```python
from build123d import *

# Parameters (mm, degrees)
SKETCH1_W                = 9
SKETCH1_H                = 55
SKETCH1_W_2              = 91
SKETCH1_H_2              = 5
BOSS_EXTRUDE3_DEPTH      = 5
SKETCH6_W                = 18
SKETCH6_H                = 60
BOSS_EXTRUDE4_DEPTH      = 18
SKETCH7_W                = 91
SKETCH7_H                = 5
BOSS_EXTRUDE5_DEPTH      = 100
SKETCH13_W               = 18
SKETCH13_H               = 5
CUT_EXTRUDE6_DEPTH       = 75
SKETCH16_R               = 4.2
CUT_EXTRUDE7_DEPTH       = 20
CUT_EXTRUDE8_DEPTH       = 75
CUT_EXTRUDE10_DEPTH      = 8
CUT_EXTRUDE11_DEPTH      = 22
CUT_EXTRUDE14_DEPTH      = 34
CUT_EXTRUDE14_DEPTH_BACK = 5
FILLET4_R                = 10
CUT_EXTRUDE15_DEPTH      = 24
CUT_EXTRUDE15_DEPTH_BACK = 1
SKETCH23_R               = 19.425
SKETCH24_R               = 1.315
CUT_EXTRUDE16_DEPTH      = 10
SKETCH26_W               = 40
SKETCH26_H               = 5
BOSS_EXTRUDE6_DEPTH      = 10


with BuildPart() as part:
    # Sketch1 → Boss-Extrude3 (new body)
    with BuildSketch(Plane.XY):
        with Locations((41, -0.737170899)):
            Rectangle(SKETCH1_W, SKETCH1_H)
        with Locations((32, -0.737170899)):
            Rectangle(SKETCH1_W, SKETCH1_H)
        with BuildLine():
            Line((27.5, 26.762829101), (0, 26.762829101))
            Line((0, 26.762829101), (0, 10.762829101))
            ThreePointArc((0, 10.762829101), (8.131727984, 7.394557085), (11.5, -0.737170899))
            ThreePointArc((11.5, -0.737170899), (8.131727984, -8.868898883), (0, -12.237170899))
            Line((0, -12.237170899), (0, -28.237170899))
            Line((0, -28.237170899), (27.5, -28.237170899))
            Line((27.5, -28.237170899), (27.5, 26.762829101))
        make_face()
        with BuildLine():
            Line((0, 10.762829101), (0, 26.762829101))
            Line((0, 26.762829101), (-27.5, 26.762829101))
            Line((-27.5, 26.762829101), (-27.5, -28.237170899))
            Line((-27.5, -28.237170899), (0, -28.237170899))
            Line((0, -28.237170899), (0, -12.237170899))
            ThreePointArc((0, -12.237170899), (-11.5, -0.737170899), (0, 10.762829101))
        make_face()
        with Locations((-32, -0.737170899)):
            Rectangle(SKETCH1_W, SKETCH1_H)
        with Locations((-41, -0.737170899)):
            Rectangle(SKETCH1_W, SKETCH1_H)
        with Locations((0, 29.262829101)):
            Rectangle(SKETCH1_W_2, SKETCH1_H_2)
    extrude(amount=BOSS_EXTRUDE3_DEPTH)

    # Sketch6 → Boss-Extrude4 (add)
    with BuildSketch(Plane(origin=(0, 0, 0), x_dir=(-1, 0, 0), z_dir=(0, 0, -1))):
        with Locations((-36.5, 1.762829101)):
            Rectangle(SKETCH6_W, SKETCH6_H)
        with Locations((36.5, 1.762829101)):
            Rectangle(SKETCH6_W, SKETCH6_H)
    extrude(amount=BOSS_EXTRUDE4_DEPTH)

    # Sketch7 → Boss-Extrude5 (add)
    with BuildSketch(Plane.XY.offset(5)):
        with Locations((0, 29.262829101)):
            Rectangle(SKETCH7_W, SKETCH7_H)
    extrude(amount=BOSS_EXTRUDE5_DEPTH)

    # Sketch13 → Cut-Extrude6 (cut)
    with BuildSketch(Plane(origin=(0, 31.762829101, 0), x_dir=(1, 0, 0), z_dir=(0, 1, 0))):
        with Locations((-36.5, 15.5)):
            Rectangle(SKETCH13_W, SKETCH13_H)
        with Locations((36.5, 15.5)):
            Rectangle(SKETCH13_W, SKETCH13_H)
    extrude(amount=-CUT_EXTRUDE6_DEPTH, mode=Mode.SUBTRACT)

    # Sketch16 → Cut-Extrude7 (cut)
    with BuildSketch(Plane(origin=(0, 31.762829101, 0), x_dir=(1, 0, 0), z_dir=(0, 1, 0))):
        with Locations(Location((-36.5, 4, 0), (0, 0, 180))):
            Circle(SKETCH16_R)
        with Locations(Location((36.5, 4, 0), (0, 0, 180))):
            Circle(SKETCH16_R)
    extrude(amount=-CUT_EXTRUDE7_DEPTH, mode=Mode.SUBTRACT)

    # Sketch17 → Cut-Extrude8 (cut)
    with BuildSketch(Plane(origin=(0, 31.762829101, 0), x_dir=(1, 0, 0), z_dir=(0, 1, 0))):
        with BuildLine():
            Line((-45.5, 13), (-45.5, 4))
            ThreePointArc((-45.5, 4), (-42.863961031, 10.363961031), (-36.5, 13))
            Line((-36.5, 13), (-45.5, 13))
        make_face()
        with BuildLine():
            ThreePointArc((-36.5, 13), (-30.136038969, 10.363961031), (-27.5, 4))
            Line((-27.5, 4), (-27.5, 13))
            Line((-27.5, 13), (-36.5, 13))
        make_face()
        with BuildLine():
            Line((27.5, 13), (27.5, 4))
            ThreePointArc((27.5, 4), (30.136038969, 10.363961031), (36.5, 13))
            Line((36.5, 13), (27.5, 13))
        make_face()
        with BuildLine():
            Line((45.5, 13), (36.5, 13))
            ThreePointArc((36.5, 13), (42.863961031, 10.363961031), (45.5, 4))
            Line((45.5, 4), (45.5, 13))
        make_face()
    extrude(amount=-CUT_EXTRUDE8_DEPTH, mode=Mode.SUBTRACT)

    # Sketch18 → Cut-Extrude10 (cut)
    with BuildSketch(Plane(origin=(0, 31.762829101, 0), x_dir=(1, 0, 0), z_dir=(0, 1, 0))):
        with BuildLine():
            ThreePointArc((-45.5, -105), (-26.743051045, -83.063543967), (-20, -55))
            Line((-20, -55), (-45.5, -55))
            Line((-45.5, -55), (-45.5, -105))
        make_face()
        with BuildLine():
            Line((-45.5, -55), (-20, -55))
            ThreePointArc((-20, -55), (-26.743051045, -26.936456033), (-45.5, -5))
            Line((-45.5, -5), (-45.5, -55))
        make_face()
        with BuildLine():
            ThreePointArc((-45.5, -105), (-26.743051045, -83.063543967), (-20, -55))
            Line((-20, -55), (-45.5, -55))
            Line((-45.5, -55), (-45.5, -105))
        make_face()
        with BuildLine():
            Line((-45.5, -55), (-20, -55))
            ThreePointArc((-20, -55), (-26.743051045, -26.936456033), (-45.5, -5))
            Line((-45.5, -5), (-45.5, -55))
        make_face()
        with BuildLine():
            Line((-20, -105), (-20, -55))
            ThreePointArc((-20, -55), (-26.743051045, -83.063543967), (-45.5, -105))
            Line((-45.5, -105), (-20, -105))
        make_face()
        with BuildLine():
            Line((20, -55), (20, -105))
            Line((20, -105), (45.5, -105))
            ThreePointArc((45.5, -105), (26.743051045, -83.063543967), (20, -55))
        make_face()
        with BuildLine():
            Line((45.5, -55), (45.5, -5))
            ThreePointArc((45.5, -5), (26.743051045, -26.936456033), (20, -55))
            Line((20, -55), (45.5, -55))
        make_face()
        with BuildLine():
            ThreePointArc((20, -55), (26.743051045, -83.063543967), (45.5, -105))
            Line((45.5, -105), (45.5, -55))
            Line((45.5, -55), (20, -55))
        make_face()
        with BuildLine():
            Line((45.5, -55), (45.5, -5))
            ThreePointArc((45.5, -5), (26.743051045, -26.936456033), (20, -55))
            Line((20, -55), (45.5, -55))
        make_face()
        with BuildLine():
            ThreePointArc((20, -55), (26.743051045, -83.063543967), (45.5, -105))
            Line((45.5, -105), (45.5, -55))
            Line((45.5, -55), (20, -55))
        make_face()
    extrude(amount=-CUT_EXTRUDE10_DEPTH, mode=Mode.SUBTRACT)

    # Sketch19 → Cut-Extrude11 (cut)
    with BuildSketch(Plane.XY.offset(5)):
        with BuildLine():
            Line((-32.5, -0.737170899), (-45.5, -0.737170899))
            Line((-45.5, -0.737170899), (-45.5, -28.237170899))
            Line((-45.5, -28.237170899), (-17.320508076, -28.237170899))
            ThreePointArc((-17.320508076, -28.237170899), (-28.453176558, -16.442798673), (-32.5, -0.737170899))
        make_face()
        with BuildLine():
            Line((45.5, -28.237170899), (17.320508076, -28.237170899))
            ThreePointArc((17.320508076, -28.237170899), (28.453176558, -16.442798673), (32.5, -0.737170899))
            Line((32.5, -0.737170899), (45.5, -0.737170899))
            Line((45.5, -0.737170899), (45.5, -28.237170899))
        make_face()
    extrude(amount=-CUT_EXTRUDE11_DEPTH, mode=Mode.SUBTRACT)

    # Sketch21 → Cut-Extrude14 (cut, two sides: drawn at the far end of the back side and taken through both)
    with BuildSketch(Plane.XZ.offset(0.737170899).offset(-CUT_EXTRUDE14_DEPTH_BACK)):
        with BuildLine():
            Line((27.5, 0), (32.5, 0))
            Line((32.5, 0), (32.5, 5))
            Line((32.5, 5), (45.5, 5))
            Line((45.5, 5), (45.5, -4))
            ThreePointArc((45.5, -4), (36.5, -13), (27.5, -4))
            Line((27.5, -4), (27.5, 0))
        make_face()
        with BuildLine():
            Line((-27.5, -4), (-27.5, 0))
            Line((-27.5, 0), (-32.5, 0))
            Line((-32.5, 0), (-32.5, 5))
            Line((-32.5, 5), (-45.5, 5))
            Line((-45.5, 5), (-45.5, -4))
            ThreePointArc((-45.5, -4), (-36.5, -13), (-27.5, -4))
        make_face()
    extrude(amount=CUT_EXTRUDE14_DEPTH + CUT_EXTRUDE14_DEPTH_BACK, mode=Mode.SUBTRACT)

    # Fillet4
    # the kernel refuses this fillet: 10 mm, written as the material it adds along each edge
    with BuildSketch(Plane(origin=(70.5, 26.762829101, 5), x_dir=(0, -1, 0), z_dir=(-1, 0, 0))) as fillet4_piece_1_section:
        with BuildLine():
            CenterArc((FILLET4_R, FILLET4_R), FILLET4_R, 180, 90)
            Line((0, FILLET4_R), (0, 0))
            Line((0, 0), (FILLET4_R, 0))
        make_face()
    fillet4_piece_1 = extrude(amount=141, mode=Mode.PRIVATE)
    fillet4_piece_1 = fillet4_piece_1 - Plane(origin=(-81.769607843, 24.471447362, 55), x_dir=(0.5871756209824568, 0, 0.8094595667010591), z_dir=(0, 1, 0)) * Cylinder(61.769607843, 322, mode=Mode.PRIVATE)
    fillet4_piece_1 = fillet4_piece_1 - Plane(origin=(81.769607843, 24.471447362, 55), x_dir=(-0.5871756209824566, 0, -0.8094595667010592), z_dir=(0, 1, 0)) * Cylinder(61.769607843, 322, mode=Mode.PRIVATE)
    add(fillet4_piece_1)

    # Sketch23 → Cut-Extrude15 (cut, two sides: drawn at the far end of the back side and taken through both)
    with BuildSketch(Plane.XY.offset(5).offset(-CUT_EXTRUDE15_DEPTH_BACK)):
        with Locations(Location((0, -0.737170899, 0), (0, 0, 115.723259522))):
            Circle(SKETCH23_R)
    extrude(amount=CUT_EXTRUDE15_DEPTH + CUT_EXTRUDE15_DEPTH_BACK, mode=Mode.SUBTRACT)

    # Sketch24 → Cut-Extrude16 (cut)
    with BuildSketch(Plane.XY.offset(4)):
        with Locations((-8.4, 13.812055885)):
            Circle(SKETCH24_R)
        with Locations((8.4, -15.286397682)):
            Circle(SKETCH24_R)
        with Locations((-8.4, -15.286397682)):
            Circle(SKETCH24_R)
        with Locations((16.8, -0.737170899)):
            Circle(SKETCH24_R)
        with Locations((-16.8, -0.737170899)):
            Circle(SKETCH24_R)
        with Locations((8.4, 13.812055885)):
            Circle(SKETCH24_R)
    extrude(amount=-CUT_EXTRUDE16_DEPTH, mode=Mode.SUBTRACT)

    # Sketch26 → Boss-Extrude6 (add)
    with BuildSketch(Plane.XY.offset(105)):
        with Locations((0, 29.262829101)):
            Rectangle(SKETCH26_W, SKETCH26_H)
    extrude(amount=BOSS_EXTRUDE6_DEPTH)


solid = part.part
```
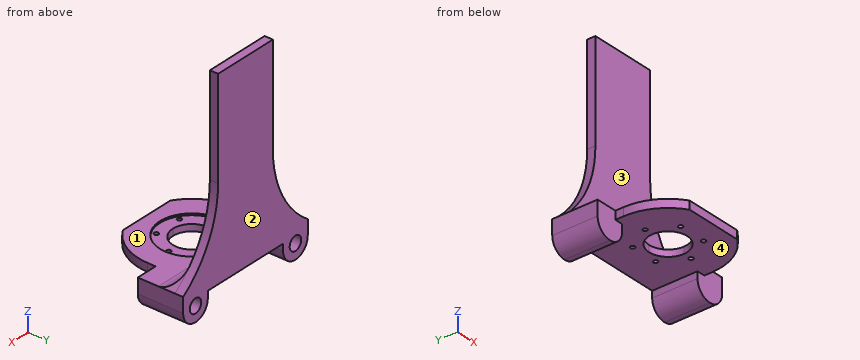
Check sheet for the modelled part. Datum: model origin and axes. Units: mm. Face numbers are marked on the shaded views. A direction names the side the tool comes from. Coordinates: 2 decimals unless noted, no trailing zeros. Loops run counter-clockwise (first coordinate to the right, second up) from the corner with the lowest first, then second, coordinate; pieces in that order, holes last.
1) Access from +Z, -Z, +X, -X, +Y, -Y to the whole of each face (thin tool, end or side, straight path). Record for the marked faces 1 and 2.
2) Sectioned sample at B-B (z = 104.5). Record the boundary of the cut face in (x, y).
3) Sectioned sample at C-C (y = 22). Record the boundary of the cut face in (x, z), and give its area (3 significant figures).
4) Release check for a two-part mould opening along X. For the marked faces 3 and 4 record: released by +X, released by -X, zero draft, split by the parting line, or undercut.
5) Gauge pin test, flat ends, axial feed: pin 1 (5 mm diameter, centred on x = -36.5, z = -4, fed in from -Y); pin 2 (2.5 mm diameter, centred on y = 2, z = 1.5, fed in from -X); pin 3 (3 mm diameter, centred on x = 4.5, y = 9.5, fed in from -Z). Record the tip position at first contact, or that the pin passes through.
6) Sectioned sample at A-A (y = 8). Record the boundary of the cut face in (x, z).
7) Material ranges on probe 1 along Y at (x, z) = (0, 4.75); probe 2 along Y at (x, z) = (16.8, 1.3); probe 3 along Z at (x, y) = (36, 16), recorded low to high.
8) Sectioned sample at D-D (y = -23). Record the boundary of the cut face in (x, z), and give its area (3 significant figures).
Check sheet entries:
1. face 1: +Z, +X, -X, -Y
1. face 2: +Z, -Z, +X, -X, +Y
2. outline: (-20, 26.76) - (20, 26.76) - (20, 31.76) - (-20, 31.76) - close
3. outline: (-45.5, -4) arc R9 ccw to (-27.5, -4) - (-27.5, 0) - (27.5, 0) - (27.5, -4) arc R9 ccw to (45.5, -4) - (45.5, 5) arc R61.77 cw to (43.54, 6.48) - (-43.54, 6.48) arc R61.77 cw to (-45.5, 5) - close; hole circle Ø8.4 at (-36.5, -4); hole circle Ø8.4 at (36.5, -4)
3. area: 874 mm2
4. face 3: zero draft
4. face 4: undercut
5. pin 1: stops at y = 4.26
5. pin 2: stops at x = -32.5
5. pin 3: stops at z = 0
6. outline: (-45.5, -4) arc R9 ccw to (-27.5, -4) - (-27.5, 0) - (-7.48, 0) - (-7.48, 4) - (-17.35, 4) - (-17.35, 5) - (-45.5, 5) - close; (7.48, 0) - (27.5, 0) - (27.5, -4) arc R9 ccw to (45.5, -4) - (45.5, 5) - (17.35, 5) - (17.35, 4) - (7.48, 4) - close
7. probe 1: y = -28.24 to -20.16, 18.69 to 31.76
7. probe 2: y = -28.24 to -2.05, 0.58 to 31.76
7. probe 3: z = -12.99 to -8.17, 0.17 to 5
8. outline: (-23.68, 0) - (23.68, 0) - (23.68, 5) - (-23.68, 5) - close
8. area: 237 mm2
